from build123d import *

# Parameters (mm, degrees)
RESSALTO_EXTRUS_O1_DEPTH = 60
ESBO_O2_R                = 25.5
CORTE_EXTRUS_O1_DEPTH    = 97.052069212
ESBO_O3_R                = 17.5
CORTE_EXTRUS_O2_DEPTH    = 97.052069212
CORTE_EXTRUS_O3_DEPTH    = 60
ESBO_O7_W                = 41
ESBO_O7_H                = 2.5
CORTE_EXTRUS_O6_DEPTH    = 50
ESBO_O6_R                = 15
CORTE_EXTRUS_O7_DEPTH    = 146.828666754
CORTE_EXTRUS_O8_DEPTH    = 53.5
CORTE_EXTRUS_O9_DEPTH    = 105.880884989
ESBO_O9_R                = 19.5
CORTE_EXTRUS_O10_DEPTH   = 146.828666754


with BuildPart() as part:
    # Esboço1 → Ressalto-extrusão1 (new body)
    with BuildSketch(Plane(origin=(0, 0, 0), x_dir=(0, 0, -1), z_dir=(1, 0, 0))):
        with BuildLine():
            Line((0, 0), (70, 0))
            Line((70, 0), (70, 5))
            ThreePointArc((70, 5), (61.782493308, 29.402148528), (59, 55))
            Line((59, 55), (51, 55))
            Line((51, 55), (51, 5))
            Line((51, 5), (0, 5))
            Line((0, 5), (0, 0))
        make_face()
    ressalto_extrus_o1 = extrude(amount=RESSALTO_EXTRUS_O1_DEPTH)

    # Esboço2 → Corte-extrusão1 (cut, through all)
    with BuildSketch(Plane.XY.offset(-51)):
        with Locations((30, 28)):
            Circle(ESBO_O2_R)
    extrude(amount=CORTE_EXTRUS_O1_DEPTH, mode=Mode.SUBTRACT)

    # Esboço3 → Corte-extrusão2 (cut, through all)
    with BuildSketch(Plane.XY.offset(-51)):
        with Locations((30, 28)):
            Circle(ESBO_O3_R)
    extrude(amount=-CORTE_EXTRUS_O2_DEPTH, mode=Mode.SUBTRACT)

    # Esboço4 → Corte-extrusão3 (cut)
    with BuildSketch(Plane.XY.offset(-51)):
        with BuildLine():
            ThreePointArc((0, 25), (8.786796564, 46.213203436), (30, 55))
            Line((30, 55), (0, 55))
            Line((0, 55), (0, 25))
        make_face()
        with BuildLine():
            Line((60, 25), (60, 55))
            Line((60, 55), (30, 55))
            ThreePointArc((30, 55), (51.213203436, 46.213203436), (60, 25))
        make_face()
    extrude(amount=-CORTE_EXTRUS_O3_DEPTH, mode=Mode.SUBTRACT)

    # Espelhar2: Ressalto-extrusão1 across plane
    add(ressalto_extrus_o1.mirror(Plane(origin=(60, 5, 0), x_dir=(1, 0, 0), z_dir=(0, 0, -1))))

    # Esboço7 → Corte-extrusão6 (cut)
    with BuildSketch(Plane(origin=(0, 55, 0), x_dir=(1, 0, 0), z_dir=(0, 1, 0))):
        with Locations((30, -52.25)):
            Rectangle(ESBO_O7_W, ESBO_O7_H)
    extrude(amount=-CORTE_EXTRUS_O6_DEPTH, mode=Mode.SUBTRACT)

    # Esboço6 → Corte-extrusão7 (cut, through all)
    with BuildSketch(Plane(origin=(0, 0, 51), x_dir=(-1, 0, 0), z_dir=(0, 0, -1))):
        with BuildLine():
            Line((-60, 55), (-60, 25))
            ThreePointArc((-60, 25), (-51.213203436, 46.213203436), (-30, 55))
            Line((-30, 55), (-60, 55))
        make_face()
        with BuildLine():
            Line((0, 55), (-30, 55))
            ThreePointArc((-30, 55), (-8.786796564, 46.213203436), (0, 25))
            Line((0, 25), (0, 55))
        make_face()
        with Locations(Location((-30, 28, 0), (0, 0, 90))):
            Circle(ESBO_O6_R)
    extrude(amount=-CORTE_EXTRUS_O7_DEPTH, mode=Mode.SUBTRACT)

    # Esboço5 → Corte-extrusão8 (cut)
    with BuildSketch(Plane(origin=(0, 0, 0), x_dir=(-1, 0, 0), z_dir=(0, 0, -1))):
        with BuildLine():
            Line((-18.988642227, 5), (-41.011357773, 5))
            ThreePointArc((-41.011357773, 5), (-30, 2.5), (-18.988642227, 5))
        make_face()
    extrude(amount=-CORTE_EXTRUS_O8_DEPTH, mode=Mode.SUBTRACT)

    # Esboço8 → Corte-extrusão9 (cut, through all)
    with BuildSketch(Plane(origin=(0, 5, 0), x_dir=(1, 0, 0), z_dir=(0, 1, 0))):
        with BuildLine():
            Line((3.5, -41), (3.5, 41))
            ThreePointArc((3.5, 41), (9.494321114, 46.994321114), (15.488642227, 41))
            Line((15.488642227, 41), (15.488642227, -41))
            ThreePointArc((15.488642227, -41), (9.494321114, -46.994321114), (3.5, -41))
        make_face()
        with BuildLine():
            Line((56.5, -41), (56.5, 41))
            ThreePointArc((56.5, 41), (50.505678886, 46.994321114), (44.511357773, 41))
            Line((44.511357773, 41), (44.511357773, -41))
            ThreePointArc((44.511357773, -41), (50.505678886, -46.994321114), (56.5, -41))
        make_face()
    extrude(amount=-CORTE_EXTRUS_O9_DEPTH, mode=Mode.SUBTRACT)

    # Esboço9 → Corte-extrusão10 (cut, through all)
    with BuildSketch(Plane.XY.offset(-51)):
        with Locations((30, 28)):
            Circle(ESBO_O9_R)
    extrude(amount=-CORTE_EXTRUS_O10_DEPTH, mode=Mode.SUBTRACT)


solid = part.part
Model file for the job. Use its own axes, mm. A direction names the side the tool comes from. Give positions to 0.01 mm unless a question says otherwise; leave off trailing zeros. Write each loop counter-clockwise with the first axis right and the second up, starting at its lowest first coordinate (ties: lowest second). Pieces come first, ordered by that corner, then holes. Notation, with made-up numbers: M 69.25,81 L 107.25,81 A26 ccw 107.25,106 Z; hole C 58,51 d6. An arc over 180 degrees is marked long. One line per item, written item: value. Start each with the question number.
Q1. Saw through at D-D, the plane x = 23. Write the cut outline in (y, z), plus the area to 3 significant figures.
Q2. Two-plate mould, pull along Z, no slides. Class faces 6 (the flat face through (30, 2, -70)), 7 (the flat face through (0, 4, -1)), 8 (the flat face through (56.5, 3, 1)), 9 (the flat face through (5, 22, 51)): +Z half, -Z half, draft (parallel to the pull), parting line (faces both ways), or undercut.
Q3. Probe probe 1 along Y at (x, z) = (30, -55.75); probe 2 along Y at (x, z) = (30, 58.75); probe 3 along Z at (x, y) = (48.5, 21.5). List the from-to ranges inside material, lowest first. Write a range as [from, to].
Q4. Saw through at B-B, the plane y = 28. Write the cut outline in (x, z), plus the area to 3 significant figures.
Q5. Saw through at A-A, the plane x = 52. Write the cut outline in (y, z).
Q6. Drop flat-ended pins along their axis: pin 1 Ø10.5 at (x, y) = (5, 28) entering from -Z; pin 2 Ø1.5 at (x, y) = (29, 41) entering from -Z; pin 3 Ø15 at (x, z) = (5, -19) entering from +Y; pin 4 Ø10.5 at (x, y) = (53.5, 28.5) entering from -Z. Give the stop position or say it passes through.
Q7. 3-axis set-ups, long thin cutter, end or side, ignore diameter. For faces 1 (the flat face through (30, 2, 70)), 2 (the flat face through (60, 4, -1)), 3 (the cylindrical face through (25.773, 8.964, -57.664)), 4 (the cylindrical face through (9.363, 2.535, -46.993)), 5 (the flat face through (9.5, 26, 52)): which of +Z, -Z, +X, -X, +Y, -Y reach the whole face in a straight line?
Q8. Saw through at C-C, the plane z = -24. Write the cut outline in (x, y), plus the area to 3 significant figures.
Output values:
1. outline: M 0,-70 L 5,-70 A119.14 cw 9.8,-67.91 L 9.8,-51 L 3.48,-51 L 3.48,53.5 L 14.73,53.5 L 14.73,66.01 A119.14 cw 5,70 L 0,70 Z; M 41.27,53.5 L 54.17,53.5 L 54.17,59 A119.14 cw 41.27,59.79 Z; M 46.2,-59.33 A119.14 cw 54.17,-59 L 54.17,-51 L 46.2,-51 Z
1. area: 907 mm²
2. face 6: -Z half
2. face 7: draft
2. face 8: undercut
2. face 9: undercut
3. probe 1: y = [0, 8.5], [47.5, 55]
3. probe 2: y = [0, 13], [43, 55]
3. probe 3: z = [-63.81, -51], [53.5, 63.81]
4. outline: M 0.15,-62.1 L 10.5,-62.1 L 10.5,-51 L 0.15,-51 Z; M 0.15,51 L 9.5,51 L 9.5,53.5 L 15,53.5 L 15,62.1 L 0.15,62.1 Z; M 45,53.5 L 50.5,53.5 L 50.5,51 L 59.85,51 L 59.85,62.1 L 45,62.1 Z; M 49.5,-62.1 L 59.85,-62.1 L 59.85,-51 L 49.5,-51 Z
4. area: 532 mm²
5. outline: M 0,-70 L 5,-70 A119.14 cw 45.4,-59.39 L 45.4,-51 L 5,-51 L 5,-46.81 L 0,-46.81 Z; M 0,46.81 L 5,46.81 L 5,51 L 45.4,51 L 45.4,59.39 A119.14 cw 5,70 L 0,70 Z
6. pin 1: stops at z = -63.45
6. pin 2: passes through
6. pin 3: stops at y = 5
6. pin 4: stops at z = -63.31
7. face 1: +Z, +X, -X, +Y, -Y
7. face 2: +Z, -Z, +X, +Y, -Y
7. face 3: -Z
7. face 4: +Y, -Y
7. face 5: +Y
8. outline: M 0,0 L 3.5,0 L 3.5,5 L 0,5 Z; M 15.49,0 L 44.51,0 L 44.51,5 L 41.01,5 A25.5 cw 18.99,5 L 15.49,5 Z; M 56.5,0 L 60,0 L 60,5 L 56.5,5 Z
8. area: 143 mm²
